```python
from build123d import *

# Parameters (mm, degrees)
SKETCH1_W               = 10.16
SKETCH1_H               = 25.4
SKETCH1_W_2             = 7.62
SKETCH1_H_2             = 22.86
BOSS_EXTRUDE1_DEPTH     = 6.35
SKETCH2_W               = 12.7
SKETCH2_H               = 27.94
SKETCH2_W_2             = 10.16
SKETCH2_H_2             = 25.4
BOSS_EXTRUDE2_DEPTH     = 1.27
SKETCH3_R               = 0.635
CUT_EXTRUDE1_DEPTH      = 11.16
CUT_EXTRUDE1_DEPTH_BACK = 3.54


with BuildPart() as part:
    # Sketch1 → Boss-Extrude1 (new body)
    with BuildSketch(Plane(origin=(0, 0, 0), x_dir=(1, 0, 0), z_dir=(0, 1, 0))):
        Rectangle(SKETCH1_W, SKETCH1_H)
        Rectangle(SKETCH1_W_2, SKETCH1_H_2, mode=Mode.SUBTRACT)
    extrude(amount=BOSS_EXTRUDE1_DEPTH)

    # Sketch2 → Boss-Extrude2 (add)
    with BuildSketch(Plane(origin=(0, 6.35, 0), x_dir=(1, 0, 0), z_dir=(0, 1, 0))):
        Rectangle(SKETCH2_W, SKETCH2_H)
        Rectangle(SKETCH2_W_2, SKETCH2_H_2, mode=Mode.SUBTRACT)
    extrude(amount=-BOSS_EXTRUDE2_DEPTH)

    # Sketch3 → Cut-Extrude1 (cut, two sides)
    with BuildSketch(Plane.ZY.offset(-3.81)) as cut_extrude1_sk:
        with Locations((0, 3.81)):
            Circle(SKETCH3_R)
    extrude(amount=CUT_EXTRUDE1_DEPTH, mode=Mode.SUBTRACT)
    extrude(cut_extrude1_sk.sketch, amount=-CUT_EXTRUDE1_DEPTH_BACK, mode=Mode.SUBTRACT)


solid = part.part
```
Source: CAD feature listing. Evaluate the final solid. Frame: model axes, mm. A direction names the side the tool comes from. Round coordinates to 2 decimals unless told otherwise and drop trailing zeros. Order: outer loops, then holes, each group sorted by start corner. A loop starts at its lowest first (then second) coordinate and runs counter-clockwise, first axis right, second up. Notation, with made-up numbers: (-32.75, 66) -> (-17.75, 66) arc R13 ccw to (-17.75, 79) -> close; hole circle Ø2 at (84.25, 20.5). An arc over 180 degrees is marked (long way). One line per item, written item: value. Start each with the question number.
Q1. Pin query (flat end, axial travel): pin 1 (2.5 mm diameter, centred on y = 3, z = 4, fed in from +X); pin 2 (2 mm diameter, centred on x = 4.5, y = 1.5, fed in from +Z); pin 3 (1.5 mm diameter, centred on y = 4, z = 7, fed in from -X). Return the tip coordinate at first contact, or that it passes through.
Q2. Draft query along Z for faces 1 (the flat face through (0, 6, 13.97)), 2 (the flat face through (-6, 5.08, -1)), 3 (the cylindrical face through (-4.44, 3.19, -0.14)). Return one class per face: pulls with the +Z half, pulls with the -Z half, needs draft (parallel to the pull), parting line crosses it, or undercut.
Q3. Section query D-D (z = 7). Return the cut outline in (x, y), plus the area to 3 significant figures.
Q4. Section query C-C (x = 0.25). Return the cut outline in (y, z), plus the area to 3 significant figures.
Q5. Access query for faces 4 (the flat face through (0, 3, 12.7)), 5 (the flat face through (0, 3, 11.43)), 6 (the flat face through (5.08, 3, 0)), 7 (the flat face through (0, 3, -12.7)). Directions: +Z, -Z, +X, -X, +Y, -Y. A direction counts if a zero-diameter tool reaches every point of the face in a straight line with its end or side. Return the directions, or none.
Q6. Material intervals for probe 1 along Y at (x, z) = (4.45, 0) (3 decimals); probe 2 along X at (y, z) = (0.5, -1.5); probe 3 along Z at (x, y) = (1.5, 3.75), sorted ascending.
Q7. Section query A-A (z = 0). Return the cut outline in (x, y) (3 decimals).
Q8. Section query B-B (y = 3.81). Return the cut outline in (x, z) (3 decimals), plus the area to 3 significant figures.
Findings below:
1. pin 1: x = 5.08
1. pin 2: z = 12.7
1. pin 3: x = -5.08
2. face 1: pulls with the +Z half
2. face 2: needs draft
2. face 3: undercut
3. outline: (-6.35, 5.08) -> (-5.08, 5.08) -> (-5.08, 0) -> (-3.81, 0) -> (-3.81, 6.35) -> (-6.35, 6.35) -> close; (3.81, 0) -> (5.08, 0) -> (5.08, 5.08) -> (6.35, 5.08) -> (6.35, 6.35) -> (3.81, 6.35) -> close
3. area: 19.4 mm²
4. outline: (0, -12.7) -> (5.08, -12.7) -> (5.08, -13.97) -> (6.35, -13.97) -> (6.35, -11.43) -> (0, -11.43) -> close; (0, 11.43) -> (6.35, 11.43) -> (6.35, 13.97) -> (5.08, 13.97) -> (5.08, 12.7) -> (0, 12.7) -> close
4. area: 19.4 mm²
5. face 4: +Z, +X, -X, -Y
5. face 5: +Y, -Y
5. face 6: +Z, -Z, +X, -Y
5. face 7: -Z, +X, -X, -Y
6. probe 1: 0 to 3.175, 4.445 to 6.35
6. probe 2: -5.08 to -3.81, 3.81 to 5.08
6. probe 3: -12.7 to -11.43, 11.43 to 12.7
7. outline: (-6.35, 5.08) -> (-5.08, 5.08) -> (-5.08, 4.445) -> (-3.81, 4.445) -> (-3.81, 6.35) -> (-6.35, 6.35) -> close; (-5.08, 0) -> (-3.81, 0) -> (-3.81, 3.175) -> (-5.08, 3.175) -> close; (3.81, 0) -> (5.08, 0) -> (5.08, 3.175) -> (3.81, 3.175) -> close; (3.81, 4.445) -> (5.08, 4.445) -> (5.08, 5.08) -> (6.35, 5.08) -> (6.35, 6.35) -> (3.81, 6.35) -> close
8. outline: (-5.08, -12.7) -> (5.08, -12.7) -> (5.08, -0.635) -> (3.81, -0.635) -> (3.81, -11.43) -> (-3.81, -11.43) -> (-3.81, -0.635) -> (-5.08, -0.635) -> close; (-5.08, 0.635) -> (-3.81, 0.635) -> (-3.81, 11.43) -> (3.81, 11.43) -> (3.81, 0.635) -> (5.08, 0.635) -> (5.08, 12.7) -> (-5.08, 12.7) -> close
8. area: 80.6 mm²
